Autodesk Inventor part; units mm, degrees
ref_plane "YZ Plane" through (0, 0, 0) normal (1, 0, 0) x (0, 1, 0)
ref_plane "XZ Plane" through (0, 0, 0) normal (0, 1, 0) x (-1, 0, 0)
ref_plane "XY Plane" through (0, 0, 0) normal (0, 0, 1) x (1, 0, 0)
sketch "Sketch1" plane through (0, 0, 0) normal (0, 0, 1) x (1, 0, 0)
  circle A0 centre (0, 0) radius 44.45
  line L0 (0, 44.45) -> (0, 69.85)
  line L1 (0, 69.85) -> (139.7, 69.85)
  line L2 (139.7, 69.85) -> (419.1, -209.55)
  line L3 (419.1, -209.55) -> (170.6858, -209.55)
  line L4 (131.4971, 12.7) -> (42.5971, 12.7)
  line L5 (131.4971, 12.7) -> (170.6858, -209.55)
  dimension "d0" = 88.9
  dimension "d1" = 25.4
  dimension "d2" = 139.7
  dimension "d3" = 88.9
  dimension "d4" = 135
  dimension "d6" = 279.4
  dimension "d7" = 0
  dimension "d8" = 12.7
  dimension "d9" = 100
extrude "Extrusion1" add sketch "Sketch1" along normal blind 9.525
properties part number "Arm"
Read the model definition and answer for the solid it produces. Units are mm, in the model's axes. A direction names the side the tool comes from. Give positions to 0.01 mm unless a question says otherwise; leave off trailing zeros. Write each loop counter-clockwise with the first axis right and the second up, starting at its lowest first coordinate (ties: lowest second). Pieces come first, ordered by that corner, then holes. Notation, with made-up numbers: (83.25, 85.5) -> (114.25, 85.5) arc R7 ccw to (114.25, 93.5) -> close; hole circle Ø11 at (-6.5, 43). An arc over 180 degrees is marked (long way). Answer as a JSON object with one key per item and string values. Group by question number.
1) Find section B-B (z = 5.5). Write down the section's boundary in (x, y).
2) Find section A-A (y = 0). Write down the section's boundary in (x, z) (3 decimals).
3) The mould has two halves that part along X. Classify faces 4 (the flat face through (277.44, -67.89, 4.7)), 5 (the flat face through (88, 12.7, 5)), 6 (the flat face through (69, 69.85, 5)): +X half, -X half, draft (parallel to the pull), parting line (faces both ways), or undercut.
4) Consider L1, parallel to Y at x = 69, z = 1.25; L2, parallel to X at y = -38.5, z = 2.5; L3, parallel to X at y = 2.5, z = 6.5. Determine where each line is inside the solid, lowest interval first. Write a range as from..to.
5) Find section C-C (x = 355.5). Write down the section's boundary in (y, z) (3 decimals).
6) Each of these flat-tipped pins is pushed along its axis until it touches: P1, Ø1, axis at y = -83, z = 5.5, coming from the -X side; P2, Ø1.5, axis at y = 38.5, z = 2.5, coming from the +X side; P3, Ø5, axis at x = 99.5, z = 4, coming from the -Y side. Where does it stop, or does it pass through?
7) Find section D-D (y = -36). Write down the section's boundary in (x, z) (3 decimals), and give its area (3 significant figures).
8) A tool of negligible diameter and unlimited length cuts with its end or side. For faces 1 (the flat face through (184, -68, 9.525)), 2 (the flat face through (0, 57, 5)), 3 (the flat face through (150.817, -96.869, 4.696)), from which of +Z, -Z, +X, -X, +Y, -Y can it reach the whole face along a straight path? Write none if from no direction.
Values follow:
{
 "1": {"outline": "(0, 44.45) arc R44.45 ccw (long way) to (42.6, 12.7) -> (131.5, 12.7) -> (170.69, -209.55) -> (419.1, -209.55) -> (139.7, 69.85) -> (0, 69.85) -> close"},
 "2": {"outline": "(-44.45, 0) -> (44.45, 0) -> (44.45, 9.525) -> (-44.45, 9.525) -> close; (133.736, 0) -> (209.55, 0) -> (209.55, 9.525) -> (133.736, 9.525) -> close"},
 "3": {"face 4": "+X half", "face 5": "undercut", "face 6": "draft"},
 "4": {"L1": "y = 12.7..69.85", "L2": "x = -22.22..22.22, 140.53..248.05", "L3": "x = -44.38..44.38, 133.3..207.05"},
 "5": {"outline": "(-209.55, 0) -> (-145.95, 0) -> (-145.95, 9.525) -> (-209.55, 9.525) -> close"},
 "6": {"P1": "stops at x = 148.28", "P2": "stops at x = 171.8", "P3": "stops at y = 12.7"},
 "7": {"outline": "(-26.073, 0) -> (26.073, 0) -> (26.073, 9.525) -> (-26.073, 9.525) -> close; (140.084, 0) -> (245.55, 0) -> (245.55, 9.525) -> (140.084, 9.525) -> close", "area": "1,500 mm2"},
 "8": {"face 1": "+Z, +X, -X, +Y, -Y", "face 2": "+Z, -Z, -X, +Y", "face 3": "+Z, -Z, -Y"}
}
